Verification items for the finished model (mm, model axes). A direction names the side the tool comes from. Coordinates: 2 decimals unless noted, no trailing zeros. Loops run counter-clockwise (first coordinate to the right, second up) from the corner with the lowest first, then second, coordinate; pieces in that order, holes last.
Q1. Sectioned sample at A-A (x = -137.1). Enter the section's corners in (y, z).
Q2. Access from +Z, -Z, +X, -X, +Y, -Y to the whole of each face (thin tool, end or side, straight path). Record for faces 4 (the face through (90.3, 0, -37)), 5 (the face through (-131.006, -8.891, -37.132)), 6 (the face through (297, 0, -59.8)), 7 (the face through (-137, 4.1, -31)), 8 (the face through (297, 0, -15)).
Q3. Sectioned sample at C-C (x = 123). Enter the section's corners in (y, z), then the cut area to 3 significant figures.
Q4. Go/stop test with flat-tipped pins: P1, Ø20, axis at y = -6, z = -19, coming from the +X side; P2, Ø1, axis at x = 291, y = -10, coming from the -Z side; P3, Ø20, axis at y = 13, z = -16.5, coming from the -X side; P4, Ø11, axis at x = -137.1, z = -37.4, coming from the +Y side. Record where each tip stops, or that it passes through.
Q5. Mould release check, pull along Y, two halves, no side actions. Record for faces 1 (the face through (297, 22.4, -38)), 2 (the face through (-130, -4.1, -38)), 3 (the face through (490.3, -12, -29)): +Y half, -Y half, draft (parallel to the pull), parting line (faces both ways), or undercut.
Q6. Material ranges on probe 1 along Y at (x, z) = (251, -35.5); probe 2 along X at (y, z) = (-11.25, -37.4); probe 3 along Z at (x, y) = (335, -1.5), recorded low to high.
Q7. Sectioned sample at B-B (x = -12.5). Enter the section's corners in (y, z).
```python
from build123d import *

# Parameters (mm, degrees)
F0_W      = 229
F0_H      = 148
F1_DEPTH  = 38
F3_DEPTH  = 35.6
F5_DEPTH  = 35
F7_D      = 12.2
F9_DEPTH  = 375.8
F11_R     = 25
F12_R     = 5
F13_DEPTH = 400
F15_DEPTH = 27.5


with BuildPart() as f1:
    # F0 (on Front) → F1 (new body, symmetric)
    with BuildSketch(Plane.XZ):
        Rectangle(F0_W, F0_H)
    extrude(amount=F1_DEPTH, both=True)

    # F2 (on face) → F3 (join)
    with BuildSketch(Plane(origin=(-114.5, 0, 0), x_dir=(0, -1, 0), z_dir=(-1, 0, 0))):
        with BuildLine():
            ThreePointArc((13.9, -37.4), (-9.8287842585, -27.5712157415), (0, -51.3))
            ThreePointArc((0, -51.3), (9.8287842585, -47.2287842585), (13.9, -37.4))
        make_face()
    extrude(amount=F3_DEPTH)

    # F4 (on face) → F5 (cut)
    with BuildSketch(Plane(origin=(-150.1, 0, 0), x_dir=(0, -1, 0), z_dir=(-1, 0, 0))):
        with BuildLine():
            ThreePointArc((13.9, -37.4), (13.8796920991, -36.6489026467), (13.8188277361, -35.9))
            Line((13.8188277361, -35.9), (13.8188277361, -38.9))
            ThreePointArc((13.8188277361, -38.9), (13.8796920991, -38.1510973533), (13.9, -37.4))
        make_face()
    extrude(amount=-F5_DEPTH, mode=Mode.SUBTRACT)

    # F7 (through all)
    with Locations(Plane.XZ.offset(13.8188277361)):
        with Locations((-137.1, -37.4)):
            Hole(F7_D / 2)

    # F8 (on face) → F9 (join)
    with BuildSketch(Plane.YZ.offset(114.5)):
        Polygon((-22.4, -59.8), (0, -59.8), (22.4, -59.8), (22.4, -15), (-22.4, -15), align=None)
    extrude(amount=F9_DEPTH)

    # F11
    f11_edges = [f1.edges().sort_by_distance(p)[0] for p in [
        (0, -38, 74),
        (0, 38, 74),
        (0, -38, -74),
        (0, 38, -74),
    ]]
    fillet(f11_edges, radius=F11_R)

    # F12
    f12_edges = [f1.edges().sort_by_distance(p)[0] for p in [
        (302.4, -22.4, -15),
        (302.4, 22.4, -15),
        (302.4, -22.4, -59.8),
        (302.4, 22.4, -59.8),
        (114.5, 38, 0),
        (-114.5, 38, 0),
        (490.3, 22.4, -37.4),
        (490.3, 0, -59.8),
        (490.3, 0, -15),
        (490.3, -22.4, -37.4),
    ]]
    fillet(f12_edges, radius=F12_R)

    # F10 (on face) → F13 (cut)
    with BuildSketch(Plane.YZ.offset(490.3)):
        with BuildLine():
            ThreePointArc((13.9, -37.4), (9.8287842585, -27.5712157415), (0, -23.5))
            ThreePointArc((0, -23.5), (-9.8287842585, -47.2287842585), (13.9, -37.4))
        make_face()
    extrude(amount=-F13_DEPTH, mode=Mode.SUBTRACT)

    # F14 (on face) → F15 (cut)
    with BuildSketch(Plane(origin=(-150.1, 0, 0), x_dir=(0, -1, 0), z_dir=(-1, 0, 0))):
        with BuildLine():
            ThreePointArc((4.1, -24.1184338273), (0, -23.5), (-4.1, -24.1184338273))
            Line((-4.1, -24.1184338273), (-4.1, -50.6815661727))
            ThreePointArc((-4.1, -50.6815661727), (-2.0731895957, -51.1445219961), (0, -51.3))
            ThreePointArc((0, -51.3), (2.0731895957, -51.1445219961), (4.1, -50.6815661727))
            Line((4.1, -50.6815661727), (4.1, -24.1184338273))
        make_face()
    extrude(amount=-F15_DEPTH, mode=Mode.SUBTRACT)


solid = f1.part
```
Geometry check:
1. outline: (-12.49, -43.5) arc R13.9 ccw to (-4.1, -50.68) - (-4.1, -43.5) - close; (-12.49, -31.3) - (-4.1, -31.3) - (-4.1, -24.12) arc R13.9 ccw to start; (4.1, -50.68) arc R13.9 ccw to (12.49, -43.5) - (4.1, -43.5) - close; (4.1, -31.3) - (12.49, -31.3) arc R13.9 ccw to (4.1, -24.12) - close
2. face 4: +X
2. face 5: +Y, -Y
2. face 6: -Z, +X, +Y, -Y
2. face 7: +Z, -Z, -X
2. face 8: +Z, +X, +Y, -Y
3. outline: (-22.4, -54.8) arc R5 ccw to (-17.4, -59.8) - (17.4, -59.8) arc R5 ccw to (22.4, -54.8) - (22.4, -20) arc R5 ccw to (17.4, -15) - (-17.4, -15) arc R5 ccw to (-22.4, -20) - close; hole circle Ø27.8 at (0, -37.4)
3. area: 1,380 mm2
4. P1: stops at x = 490.3
4. P2: stops at z = -59.8
4. P3: stops at x = -114.5
4. P4: passes through
5. face 1: +Y half
5. face 2: undercut
5. face 3: draft
6. probe 1: y = -22.4 to -13.77, 13.77 to 22.4
6. probe 2: x = -150.1 to -143.2, -131 to 90.3
6. probe 3: z = -59.8 to -51.22, -23.58 to -15
7. outline: (-38, -49) arc R25 ccw to (-13, -74) - (13, -74) arc R25 ccw to (38, -49) - (38, 49) arc R25 ccw to (13, 74) - (-13, 74) arc R25 ccw to (-38, 49) - close
